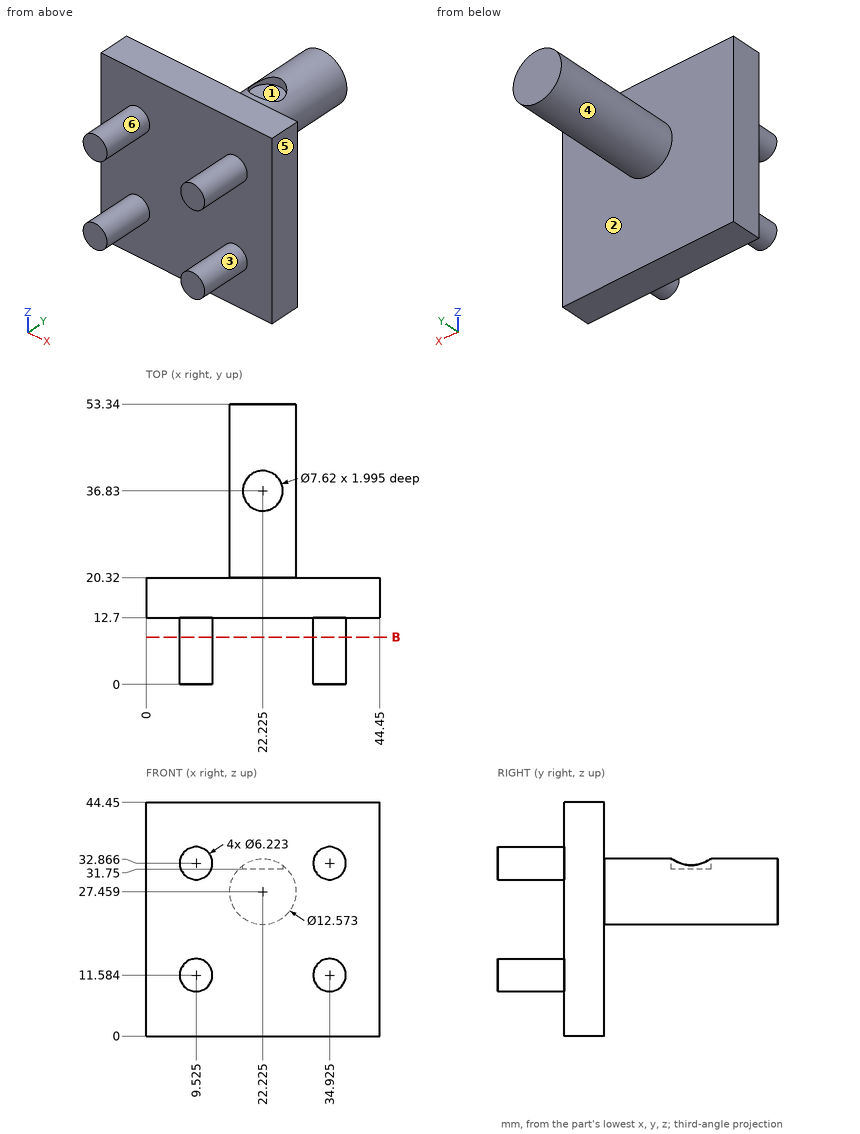
Drawing for the job (mm, zero at the part's lowest x, y, z). A direction names the side the tool comes from. Round coordinates to 2 decimals unless told otherwise and drop trailing zeros. Write each loop counter-clockwise with the first axis right and the second up, starting at its lowest first coordinate (ties: lowest second). Pieces come first, ordered by that corner, then holes. Notation, with made-up numbers: M 74.25,25 L 115.25,25 A16 cw 115.25,30 Z; hole C -18.5,44 d11. An arc over 180 degrees is marked long. One line per question, with ' | ' between items.
1. Mould opens along Z. For the marked faces 1, 2, 3 and 4 say: pulls with the +Z half, pulls with the -Z half, needs draft (parallel to the pull), parting line crosses it, or undercut.
Working result:
face 1: pulls with the +Z half | face 2: needs draft | face 3: undercut | face 4: parting line crosses it
2. Probe L1, parallel to Y at x = 17, z = 27; L2, parallel to Y at x = 24, z = 17; L3, parallel to Z at x = 36.5, y = 2. List the from-to ranges inside material, lowest first. Write a range as from..to.
Working result:
L1: 12.7..53.34 | L2: 12.7..20.32 | L3: 8.9..14.27, 30.18..35.55
3. Pin check, flat tips, straight feed: pin 1 Ø1 at (x, y) = (36, 12) entering from -Z; pin 2 Ø2 at (x, y) = (20.5, 46) entering from -Z; pin 3 Ø12 at (x, y) = (22.225, 36.83) entering from +Z (1 decimal); pin 4 Ø8 at (x, y) = (35, 31) entering from -Z. Stop position of each tip, or through.
Working result:
pin 1: z = 8.53 | pin 2: z = 21.21 | pin 3: z = 33.7 | pin 4: through
4. Cut at B-B on y = 9. Write the cut outline in (x, z) (1 decimal), and give its area (3 significant figures).
Working result:
outline: C 9.5,11.6 d6.2; C 9.5,32.9 d6.2; C 34.9,11.6 d6.2; C 34.9,32.9 d6.2 | area: 122 mm2
5. Which spindle directions (+Z, -Z, +X, -X, +Y, -Y) get a long thin tool onto all of the face, cutting with end or side? Do the marked faces 5 and 6. Say none if no direction does.
Working result:
face 5: +Z, -Z, +X, +Y, -Y | face 6: -Y
